from build123d import *

# Parameters (mm, degrees)
SZKIC1_R                    = 75
DODANIE_WYCI_GNI_CIE1_DEPTH = 20
SZKIC2_R                    = 14
DODANIE_WYCI_GNI_CIE2_DEPTH = 20
SZKIC3_R                    = 7
DODANIE_WYCI_GNI_CIE3_DEPTH = 6
DODANIE_WYCI_GNI_CIE4_DEPTH = 25
SFAZOWANIE1_SIZE            = 5
SZKIC5_R                    = 17.5
DODANIE_WYCI_GNI_CIE5_DEPTH = 114
OTW_R_POD_RUB_M41_D         = 4.5


with BuildPart() as part:
    # Szkic1 → Dodanie-wyciągnięcie1 (new, symmetric)
    with BuildSketch(Plane(origin=(0, 0, 0), x_dir=(0, 0, -1), z_dir=(1, 0, 0))):
        Circle(SZKIC1_R)
    extrude(amount=DODANIE_WYCI_GNI_CIE1_DEPTH, both=True)

    # Szkic2 → Dodanie-wyciągnięcie2 (add)
    with BuildSketch(Plane.ZY.offset(20)):
        Circle(SZKIC2_R)
    extrude(amount=DODANIE_WYCI_GNI_CIE2_DEPTH)

    # Szkic3 → Dodanie-wyciągnięcie3 (add)
    with BuildSketch(Plane.ZY.offset(40)):
        Circle(SZKIC3_R)
    extrude(amount=DODANIE_WYCI_GNI_CIE3_DEPTH)

    # Szkic4 → Dodanie-wyciągnięcie4 (add, symmetric)
    with BuildSketch(Plane.XY):
        Polygon((-46, -20), (-46, 30), (-104, 30), (-104, -20), (-97, -20), (-97, 22), (-58, 22), (-58, -20), align=None)
    extrude(amount=DODANIE_WYCI_GNI_CIE4_DEPTH, both=True)

    # Sfazowanie1
    sfazowanie1_edges = [part.edges().sort_by_distance(p)[0] for p in [
        (-97, 22, 0),
        (-58, 22, 0),
    ]]
    chamfer(sfazowanie1_edges, length=SFAZOWANIE1_SIZE)

    # Szkic5 → Dodanie-wyciągnięcie5 (add)
    with BuildSketch(Plane.ZY.offset(104)):
        with Locations(Location((0, 0, 0), (0, 0, 180))):
            Circle(SZKIC5_R)
    extrude(amount=DODANIE_WYCI_GNI_CIE5_DEPTH)

    # Otwór pod śrubę M41 (through all)
    with Locations(Plane(origin=(0, 30, 0), x_dir=(1, 0, 0), z_dir=(0, 1, 0))):
        with Locations((-68, 18), (-86, 18), (-68, -18), (-86, -18)):
            Hole(OTW_R_POD_RUB_M41_D / 2)


solid = part.part
The model under review builds one solid part; all positions refer to its coordinate system, in mm. A direction names the side the tool comes from. Give positions to 0.01 mm unless a question says otherwise; leave off trailing zeros. Order: outer loops, then holes, each group sorted by start corner. A loop starts at its lowest first (then second) coordinate and runs counter-clockwise, first axis right, second up. Notation, with made-up numbers: M 86.5,62.25 L 130.5,62.25 A22 ccw 130.5,82.25 Z; hole C 52,77.5 d2. An arc over 180 degrees is marked long. Use one line per item in the form item = value. Start each with the question number.
Item 1: Insertion check: pin 1 Ø9.5 at (x, z) = (-53, -1.5) entering from -Y; pin 2 Ø7 at (x, z) = (-86, -18) entering from +Y; pin 3 Ø8.5 at (x, z) = (-79, 1) entering from -Y; pin 4 Ø3.5 at (x, z) = (-86, 18) entering from -Y. Each pin has a flat end and moves straight along its axis. Give the tip position at first contact, or say it passes through.
Item 2: For faces 1 (the flat face through (-101, -20, 0)), 2 (the flat face through (-40, 3.3, -6.4)), 3 (the flat face through (-94, 20, 0)), 4 (the flat face through (-62.5, 22, -25)), list the 3-axis set-ups (+Z, -Z, +X, -X, +Y, -Y) from which the entire face can be reached by the end or side of a thin tool; tool diameter is ignored.
Item 3: We need section B-B on z = 0. Give the boundary of the cut face in (x, y).
Item 4: We need section A-A on y = 0. Give the boundary of the cut face in (x, z), plus the area to 3 significant figures.
Item 5: The part is to be moulded in two halves that separate along X. For faces 5 (the cylindrical face through (-29.86, -5.362, 12.932)), 6 (the cylindrical face through (-160.202, 17.084, 3.794)), 7 (the flat face through (-46, 10, 0)), 8 (the flat face through (-104, 16, 11)), say which applies: pulls with the +X half, pulls with the -X half, needs draft (parallel to the pull), parting line crosses it, or undercut.
Item 6: We need section D-D on y = -58. Give the boundary of the cut face in (x, z), plus the area to 3 significant figures.
Item 7: We need section C-C on x = -150. Give the boundary of the cut face in (y, z), plus the area to 3 significant figures.
Item 8: To check wall thickness, follow line 1 along X through (y, z) = (26, -18); line 2 along X through (y, z) = (-10.5, -9.5); line 3 along Z through (x, y) = (-86, 25). State the ranges of each line that lie inside material, in increasing order. Write a range as from..to.
Completed:
q1.pin_1 = -20
q1.pin_2 = 30
q1.pin_3 = 22
q1.pin_4 = through
q2.face_1 = +Z, -Z, -X, -Y
q2.face_2 = none
q2.face_3 = +Z, -Z, -Y
q2.face_4 = -Z, -X, +Y, -Y
q3.outline = M -218,-17.5 L -104,-17.5 L -104,-20 L -97,-20 L -97,17 L -92,22 L -63,22 L -58,17 L -58,-20 L -46,-20 L -46,-7 L -40,-7 L -40,-14 L -20,-14 L -20,-75 L 20,-75 L 20,75 L -20,75 L -20,14 L -40,14 L -40,7 L -46,7 L -46,30 L -104,30 L -104,17.5 L -218,17.5 Z
q4.outline = M -218,-17.5 L -104,-17.5 L -104,-25 L -97,-25 L -97,25 L -104,25 L -104,17.5 L -218,17.5 Z; M -58,-25 L -46,-25 L -46,-7 L -40,-7 L -40,-14 L -20,-14 L -20,-75 L 20,-75 L 20,75 L -20,75 L -20,14 L -40,14 L -40,7 L -46,7 L -46,25 L -58,25 Z
q4.area = 11,600 mm²
q5.face_5 = undercut
q5.face_6 = needs draft
q5.face_7 = undercut
q5.face_8 = pulls with the -X half
q6.outline = M -20,-47.55 L 20,-47.55 L 20,47.55 L -20,47.55 Z
q6.area = 3,800 mm²
q7.outline = C 0,0 d35
q7.area = 962 mm²
q8.line_1 = -104..-88.25, -83.75..-70.25, -65.75..-46, -20..20
q8.line_2 = -218..-97, -58..-46, -20..20
q8.line_3 = -25..-20.25, -15.75..15.75, 20.25..25
